Can you work these out from the model? Positions are in its coordinate system, mm. A direction names the side the tool comes from. Round coordinates to 2 decimals unless told otherwise and drop trailing zeros. Order: outer loops, then holes, each group sorted by start corner. A loop starts at its lowest first (then second) coordinate and runs counter-clockwise, first axis right, second up.
from build123d import *

# Parameters (mm, degrees)
F1_DEPTH = 203.2
F2_R     = 38.1
F3_DEPTH = 76.2
F5_DEPTH = 50.8


with BuildPart() as f1:
    # F0 (on Front) → F1 (new body)
    with BuildSketch(Plane.XZ):
        Polygon((-254, 0), (0, 0), (0, 50.8), (-125.723586, 176.523586), (-176.523586, 125.723586), (-101.6, 50.8), (-254, 50.8), align=None)
    extrude(amount=-F1_DEPTH)

    # F2 (on face) → F3 (cut)
    with BuildSketch(Plane(origin=(25.4, 0, 25.4), x_dir=(0.707107, 0, -0.707107), z_dir=(0.707107, 0, 0.707107))):
        with Locations((-162.921024, 101.6)):
            Circle(F2_R)
    extrude(amount=-F3_DEPTH, mode=Mode.SUBTRACT)

    # F4 (on face) → F5 (cut)
    with BuildSketch(Plane.XY.offset(50.8)):
        Polygon((-254, 203.2), (-254, 152.4), (-203.2, 203.2), align=None)
        Polygon((-254, 50.8), (-254, 0), (-203.2, 0), align=None)
    extrude(amount=-F5_DEPTH, mode=Mode.SUBTRACT)


solid = f1.part
(1) I want a section at A-A, the plane y = 84.5. List the corners of the cut face in (x, z) for me, plus the area to 3 significant figures.
(2) On a 3-axis mill with a long thin cutter (end or side, diameter ignored), from which of +Z, -Z, +X, -X, +Y, -Y can I reach the whole of each face in a straight line? I mean faces 1 (the face through (-129, 100, 0)), 2 (the face through (-177, 100, 50.8)). Say none if no direction works.
(3) I'm going to push flat-ended pins straight in: pin 1 Ø12 at (x, y) = (-178, 36.5) entering from +Z; pin 2 Ø12 at (x, y) = (-133.5, 56.5) entering from +Z; pin 3 Ø12 at (y, z) = (46.5, 148) entering from -X. Where does each tip first touch, or does it pass through?
(4) I want a section at C-C, the plane y = 168. List the corners of the cut face in (x, z) for me, plus the area to 3 significant figures.
(5) I want a section at D-D, the plane x = -38. List the corners of the cut face in (y, z) for me, plus the area to 3 significant figures.
(6) If we mould it in two halves opening along Z, with no side actions, what happens to faces 3 (the face through (-136.23, 78.42, 136.94)), 4 (the face through (-254, 101, 26)), 5 (the face through (-62, 100.2, 112.8)), 6 (the face through (-164.6, 77.6, 113.8))? For each: pulls with the +Z half, pulls with the -Z half, needs draft (parallel to the pull), parting line crosses it, or undercut.
(7) Please list where these lines run through material, in increasing order: probe 1 along Z at (x, y) = (-126.5, 188.5); probe 2 along Z at (x, y) = (-192.5, 55.5); probe 3 along Z at (x, y) = (-106, 81).
(8) I want a section at B-B, the plane z = 44. List the corners of the cut face in (x, y) for me.
Ans:
1. outline: (-254, 0) - (0, 0) - (0, 50.8) - (-65.73, 116.53) - (-116.53, 65.73) - (-101.6, 50.8) - (-254, 50.8) - close; (-176.52, 125.72) - (-164.68, 113.88) - (-113.88, 164.68) - (-125.72, 176.52) - close
1. area: 18,200 mm2
2. face 1: -Z, +X, -X, +Y, -Y
2. face 2: -X, +Y, -Y
3. pin 1: stops at z = 130.25
3. pin 2: stops at z = 174.75
3. pin 3: stops at x = -160.25
4. outline: (-238.4, 0) - (0, 0) - (0, 50.8) - (-125.72, 176.52) - (-176.52, 125.72) - (-101.6, 50.8) - (-238.4, 50.8) - close
4. area: 22,300 mm2
5. outline: (0, 0) - (203.2, 0) - (203.2, 88.8) - (0, 88.8) - close
5. area: 18,000 mm2
6. face 3: undercut
6. face 4: needs draft
6. face 5: pulls with the +Z half
6. face 6: undercut
7. probe 1: z = 0 to 50.8, 75.7 to 175.75
7. probe 2: z = 0 to 50.8
7. probe 3: z = 0 to 50.8, 55.2 to 79.08
8. outline: (-254, 50.8) - (-203.2, 0) - (0, 0) - (0, 203.2) - (-203.2, 203.2) - (-254, 152.4) - close
